Geometry: see drawing. Coordinates: mm, zero at the bounding-box minimum. Coordinates: 2 decimals unless noted, no trailing zeros. Order: outer loops, then holes, each group sorted by start corner. A loop starts at its lowest first (then second) coordinate and runs counter-clockwise, first axis right, second up.
Item 1: Section B-B on x = 125.2. Return the cut outline in (y, z).
Item 2: Ray query, line 1 (Y direction, x = 90, z = 4.25); line 2 (X direction, y = 7.25, z = 1.5); line 3 (Y direction, x = 91.5, z = 8). Return the intervals inside material, ascending.
Item 3: Section A-A on y = 12.5. Return the cut outline in (x, z), then the cut area to 3 significant figures.
Item 4: Section D-D on z = 9.75. Return the cut outline in (x, y), then the cut area to 3 significant figures.
Item 5: Section C-C on x = 45. Return the cut outline in (y, z), then the cut area to 3 significant figures.
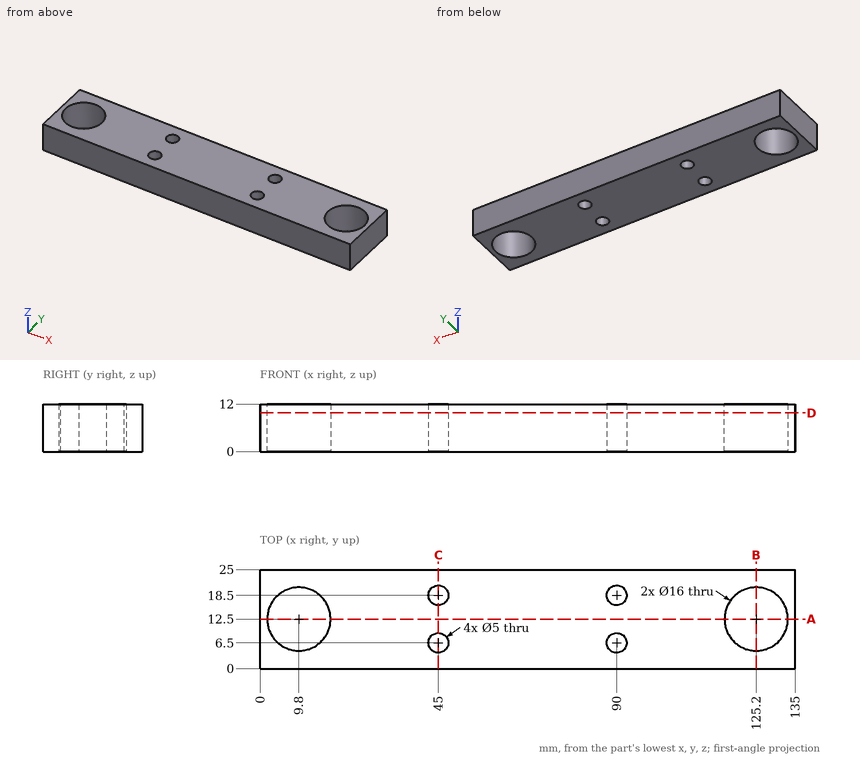
Answer list:
1. outline: (0, 0) - (4.5, 0) - (4.5, 12) - (0, 12) - close; (20.5, 0) - (25, 0) - (25, 12) - (20.5, 12) - close
2. line 1: y = 0 to 4, 9 to 16, 21 to 25
2. line 2: x = 0 to 3.76, 15.84 to 42.62, 47.38 to 87.62, 92.38 to 119.16, 131.24 to 135
2. line 3: y = 0 to 4.5, 8.5 to 16.5, 20.5 to 25
3. outline: (0, 0) - (1.8, 0) - (1.8, 12) - (0, 12) - close; (17.8, 0) - (117.2, 0) - (117.2, 12) - (17.8, 12) - close; (133.2, 0) - (135, 0) - (135, 12) - (133.2, 12) - close
3. area: 1,240 mm2
4. outline: (0, 0) - (135, 0) - (135, 25) - (0, 25) - close; hole circle Ø16 at (9.8, 12.5); hole circle Ø5 at (45, 6.5); hole circle Ø5 at (45, 18.5); hole circle Ø5 at (90, 6.5); hole circle Ø5 at (90, 18.5); hole circle Ø16 at (125.2, 12.5)
4. area: 2,890 mm2
5. outline: (0, 0) - (4, 0) - (4, 12) - (0, 12) - close; (9, 0) - (16, 0) - (16, 12) - (9, 12) - close; (21, 0) - (25, 0) - (25, 12) - (21, 12) - close
5. area: 180 mm2
